from build123d import *

# Parameters (mm, degrees)
BOX002_W            = 5
BOX002_H            = 1
BOX002_DEPTH        = 5
BOX001_W            = 5
BOX001_H            = 1
BOX001_DEPTH        = 5
CYLINDER_R          = 5
CYLINDER_DEPTH      = 2
CYLINDER_ROLL_ANGLE = 90
BOX_W               = 10
BOX_H               = 20
BOX_DEPTH           = 8


with BuildPart() as interior_opening:
    # Box002 → Box002 (new body)
    with BuildSketch(Plane(origin=(2.5, 3, 3), x_dir=(1, 0, 0), z_dir=(0, 0, 1))):
        with Locations((2.5, 0.5)):
            Rectangle(BOX002_W, BOX002_H)
    extrude(amount=BOX002_DEPTH)


with BuildPart() as end_opening:
    # Box001 → Box001 (new body)
    with BuildSketch(Plane(origin=(2.5, 0, 3), x_dir=(1, 0, 0), z_dir=(0, 0, 1))):
        with Locations((2.5, 0.5)):
            Rectangle(BOX001_W, BOX001_H)
    extrude(amount=BOX001_DEPTH)


with BuildPart() as solenoid_head_slot:
    # Cylinder → Cylinder (new body)
    with BuildSketch(Plane.XY):
        Circle(CYLINDER_R)
    extrude(amount=CYLINDER_DEPTH)


with BuildPart() as solenoid_head_slot_1:
    # Cylinder roll: moved
    add(solenoid_head_slot.part.rotate(Axis((0, 0, 0), (1, 0, 0)), CYLINDER_ROLL_ANGLE))


with BuildPart() as solenoid_head_slot_2:
    # Cylinder placement: moved
    add(solenoid_head_slot_1.part.moved(Location((5, 3, 5))))


with BuildPart() as cut002:
    # Box → Box (new body)
    with BuildSketch(Plane.XY):
        with Locations((5, 10)):
            Rectangle(BOX_W, BOX_H)
    extrude(amount=BOX_DEPTH)

    # Cut: cut solenoid_head_slot
    add(solenoid_head_slot_2.part, mode=Mode.SUBTRACT)

    # Cut001: cut end_opening
    add(end_opening.part, mode=Mode.SUBTRACT)

    # Cut002: cut interior_opening
    add(interior_opening.part, mode=Mode.SUBTRACT)


solid = cut002.part
Design review of the part built by this model. Coordinates are the model's own, in mm. A direction names the side the tool comes from. Coordinates: 2 decimals unless noted, no trailing zeros. Write each loop counter-clockwise with the first axis right and the second up, starting at its lowest first coordinate (ties: lowest second). Pieces come first, ordered by that corner, then holes. Notation, with made-up numbers: (4, 8) -> (60, 8) arc R28 ccw to (60, 40) -> close; hole circle Ø5 at (77, 13.25). An arc over 180 degrees is marked (long way). Write each question's results on one line, items separated by ' | '. Start each with the question number.
(1) The part is to be moulded in two halves that separate along Y. For faces 4 (the face through (5, 4, 5)), 5 (the face through (7.5, 3.5, 5.5)), 6 (the face through (9.75, 2.01, 6.56)), say which applies: pulls with the +Y half, pulls with the -Y half, needs draft (parallel to the pull), parting line crosses it, or undercut.
(2) Take a section at A-A on z = 1. Write out the cut boundary in (x, y).
(3) Take a section at B-B on y = 3.5. Write out the cut boundary in (x, z), and give its area (3 significant figures).
(4) Take a section at C-C on x = 5.5. Write out the cut boundary in (y, z), and give its area (3 significant figures).
(5) For line 1 along X through (y, z) = (3.75, 4); line 2 along Y through (x, z) = (3.75, 1.5); line 3 along Y through (x, z) = (7.25, 3.75), list the stretches that pass through material, from the lowest coordinate up. Write a range as from..to.
(6) Clearance check with flat-ended pins moving along their axes: P1, Ø0.5, axis at x = 4, y = 0.5, coming from the +Z side; P2, Ø1, axis at x = 7.5, y = 12, coming from the -Z side. State where each tip first meets the part, or that it passes through.
(7) Take a section at D-D on z = 5.75. Write out the cut boundary in (x, y).
(8) Tool access review of faces 1 (the face through (5, 0.5, 3)), 2 (the face through (0, 10, 4)), 3 (the face through (1, 2, 2)): name each direction out of +Z, -Z, +X, -X, +Y, -Y from which nothing blocks a thin tool from reaching the whole face with its end or side.
Results found:
1) face 4: pulls with the -Y half | face 5: needs draft | face 6: undercut
2) outline: (0, 0) -> (10, 0) -> (10, 20) -> (0, 20) -> close; hole (2, 1) -> (8, 1) -> (8, 3) -> (2, 3) -> close
3) outline: (0, 0) -> (10, 0) -> (10, 8) -> (7.5, 8) -> (7.5, 3) -> (2.5, 3) -> (2.5, 8) -> (0, 8) -> close | area: 55.0 mm2
4) outline: (0, 0) -> (20, 0) -> (20, 8) -> (4, 8) -> (4, 3) -> (3, 3) -> (3, 0.03) -> (1, 0.03) -> (1, 3) -> (0, 3) -> close | area: 134 mm2
5) line 1: x = 0..2.5, 7.5..10 | line 2: y = 0..1, 3..20 | line 3: y = 4..20
6) P1: stops at z = 3 | P2: stops at z = 0
7) outline: (0, 0) -> (2.5, 0) -> (2.5, 1) -> (0.06, 1) -> (0.06, 3) -> (2.5, 3) -> (2.5, 4) -> (7.5, 4) -> (7.5, 3) -> (9.94, 3) -> (9.94, 1) -> (7.5, 1) -> (7.5, 0) -> (10, 0) -> (10, 20) -> (0, 20) -> close
8) face 1: +Z, -Y | face 2: +Z, -Z, -X, +Y, -Y | face 3: none
